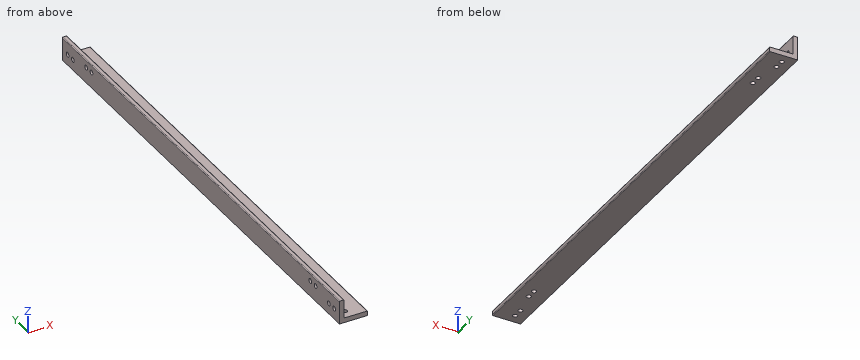
from build123d import *

# Parameters (mm, degrees)
SKETCH1_W           = 15
SKETCH1_H           = 313
SKETCH1_R           = 1.5
BOSS_EXTRUDE2_DEPTH = 3
SKETCH1_4_W         = 3
SKETCH1_4_H         = 313
BOSS_EXTRUDE3_DEPTH = 15
CUT_EXTRUDE1_REACH  = 20
SKETCH2_R           = 1.5
FILLET1_R           = 0.5


with BuildPart() as part:
    # Sketch1 → Boss-Extrude2 (new body)
    with BuildSketch(Plane.XY):
        with Locations((7.842857143, -137.142857143)):
            Rectangle(SKETCH1_W, SKETCH1_H)
        with Locations((4.142857143, 13.357142857)):
            Circle(SKETCH1_R, mode=Mode.SUBTRACT)
        with Locations((4.142857143, -287.642857143)):
            Circle(SKETCH1_R, mode=Mode.SUBTRACT)
        with Locations((4.142857143, 7.357142857)):
            Circle(SKETCH1_R, mode=Mode.SUBTRACT)
        with Locations((4.142857143, -281.642857143)):
            Circle(SKETCH1_R, mode=Mode.SUBTRACT)
        with Locations((7.342857143, -266.642857143)):
            Circle(SKETCH1_R, mode=Mode.SUBTRACT)
        with Locations((7.342857143, -260.642857143)):
            Circle(SKETCH1_R, mode=Mode.SUBTRACT)
        with Locations((7.342857143, -13.642857143)):
            Circle(SKETCH1_R, mode=Mode.SUBTRACT)
        with Locations((7.342857143, -7.642857143)):
            Circle(SKETCH1_R, mode=Mode.SUBTRACT)
    extrude(amount=BOSS_EXTRUDE2_DEPTH)

    # Sketch1_4 → Boss-Extrude3 (add)
    with BuildSketch(Plane.XY):
        with Locations((-1.157142857, -137.142857143)):
            Rectangle(SKETCH1_4_W, SKETCH1_4_H)
    extrude(amount=BOSS_EXTRUDE3_DEPTH)

    # Sketch2 → Cut-Extrude1 (cut, up to next)
    with BuildSketch(Plane.ZY.offset(2.657142857), mode=Mode.PRIVATE) as cut_extrude1_sk1:
        with Locations((6.8, 13.357142857)):
            Circle(SKETCH2_R)
    cut_extrude1_tool1 = extrude(cut_extrude1_sk1.sketch, amount=-CUT_EXTRUDE1_REACH, mode=Mode.PRIVATE) & part.part
    add(cut_extrude1_tool1.solids().sort_by_distance((-2.657143, 13.357143, 6.8))[0], mode=Mode.SUBTRACT)
    # Sketch2 → Cut-Extrude1 (cut, up to next)
    with BuildSketch(Plane.ZY.offset(2.657142857), mode=Mode.PRIVATE) as cut_extrude1_sk2:
        with Locations((6.8, -287.642857143)):
            Circle(SKETCH2_R)
    cut_extrude1_tool2 = extrude(cut_extrude1_sk2.sketch, amount=-CUT_EXTRUDE1_REACH, mode=Mode.PRIVATE) & part.part
    add(cut_extrude1_tool2.solids().sort_by_distance((-2.657143, -287.642857, 6.8))[0], mode=Mode.SUBTRACT)
    # Sketch2 → Cut-Extrude1 (cut, up to next)
    with BuildSketch(Plane.ZY.offset(2.657142857), mode=Mode.PRIVATE) as cut_extrude1_sk3:
        with Locations((6.8, -281.642857143)):
            Circle(SKETCH2_R)
    cut_extrude1_tool3 = extrude(cut_extrude1_sk3.sketch, amount=-CUT_EXTRUDE1_REACH, mode=Mode.PRIVATE) & part.part
    add(cut_extrude1_tool3.solids().sort_by_distance((-2.657143, -281.642857, 6.8))[0], mode=Mode.SUBTRACT)
    # Sketch2 → Cut-Extrude1 (cut, up to next)
    with BuildSketch(Plane.ZY.offset(2.657142857), mode=Mode.PRIVATE) as cut_extrude1_sk4:
        with Locations((6.8, 7.357142857)):
            Circle(SKETCH2_R)
    cut_extrude1_tool4 = extrude(cut_extrude1_sk4.sketch, amount=-CUT_EXTRUDE1_REACH, mode=Mode.PRIVATE) & part.part
    add(cut_extrude1_tool4.solids().sort_by_distance((-2.657143, 7.357143, 6.8))[0], mode=Mode.SUBTRACT)
    # Sketch2 → Cut-Extrude1 (cut, up to next)
    with BuildSketch(Plane.ZY.offset(2.657142857), mode=Mode.PRIVATE) as cut_extrude1_sk5:
        with Locations((10, -266.642857143)):
            Circle(SKETCH2_R)
    cut_extrude1_tool5 = extrude(cut_extrude1_sk5.sketch, amount=-CUT_EXTRUDE1_REACH, mode=Mode.PRIVATE) & part.part
    add(cut_extrude1_tool5.solids().sort_by_distance((-2.657143, -266.642857, 10))[0], mode=Mode.SUBTRACT)
    # Sketch2 → Cut-Extrude1 (cut, up to next)
    with BuildSketch(Plane.ZY.offset(2.657142857), mode=Mode.PRIVATE) as cut_extrude1_sk6:
        with Locations((10, -260.642857143)):
            Circle(SKETCH2_R)
    cut_extrude1_tool6 = extrude(cut_extrude1_sk6.sketch, amount=-CUT_EXTRUDE1_REACH, mode=Mode.PRIVATE) & part.part
    add(cut_extrude1_tool6.solids().sort_by_distance((-2.657143, -260.642857, 10))[0], mode=Mode.SUBTRACT)
    # Sketch2 → Cut-Extrude1 (cut, up to next)
    with BuildSketch(Plane.ZY.offset(2.657142857), mode=Mode.PRIVATE) as cut_extrude1_sk7:
        with Locations((10, -13.642857143)):
            Circle(SKETCH2_R)
    cut_extrude1_tool7 = extrude(cut_extrude1_sk7.sketch, amount=-CUT_EXTRUDE1_REACH, mode=Mode.PRIVATE) & part.part
    add(cut_extrude1_tool7.solids().sort_by_distance((-2.657143, -13.642857, 10))[0], mode=Mode.SUBTRACT)
    # Sketch2 → Cut-Extrude1 (cut, up to next)
    with BuildSketch(Plane.ZY.offset(2.657142857), mode=Mode.PRIVATE) as cut_extrude1_sk8:
        with Locations((10, -7.642857143)):
            Circle(SKETCH2_R)
    cut_extrude1_tool8 = extrude(cut_extrude1_sk8.sketch, amount=-CUT_EXTRUDE1_REACH, mode=Mode.PRIVATE) & part.part
    add(cut_extrude1_tool8.solids().sort_by_distance((-2.657143, -7.642857, 10))[0], mode=Mode.SUBTRACT)

    # Fillet1
    fillet1_edges = [part.edges().sort_by_distance(p)[0] for p in [
        (15.342857143, -137.142857143, 0),
        (0.342857143, -137.142857143, 15),
        (-2.657142857, -137.142857143, 15),
        (15.342857143, -137.142857143, 3),
        (0.342857143, -137.142857143, 3),
    ]]
    fillet(fillet1_edges, radius=FILLET1_R)


solid = part.part
Part model, mm, in its own coordinate system. Coordinates: 2 decimals unless noted, no trailing zeros. Write each loop counter-clockwise with the first axis right and the second up, starting at its lowest first coordinate (ties: lowest second). Pieces come first, ordered by that corner, then holes. Notation, with made-up numbers: M -21.75,56 L 19.25,56 A17 ccw 19.25,83 Z; hole C -29.75,48.25 d1. An arc over 180 degrees is marked long. Return JSON: item names as keys, results as strings.
1. Probe L1, parallel to Y at x = -1.7, z = 10; L2, parallel to Y at x = 6.75, z = 0.5; L3, parallel to X at y = -264.5, z = 10. List the from-to ranges inside material, lowest first.
Determined:
{"L1": "-293.64 to -268.14, -265.14 to -262.14, -259.14 to -15.14, -12.14 to -9.14, -6.14 to 19.36", "L2": "-293.64 to -268.02, -265.26 to -262.02, -259.26 to -15.02, -12.26 to -9.02, -6.26 to 19.36", "L3": "-2.66 to 0.34"}
2. Saw through at A-A, the plane y = -147. Write the cut outline in (x, z), then the cut area to 3 significant figures.
Determined:
{"outline": "M -2.66,0 L 14.84,0 A0.5 ccw 15.34,0.5 L 15.34,2.5 A0.5 ccw 14.84,3 L 0.84,3 A0.5 cw 0.34,3.5 L 0.34,14.5 A0.5 ccw -0.16,15 L -2.16,15 A0.5 ccw -2.66,14.5 Z", "area": "89.8 mm²"}
3. Flat gauge pins, fed straight in: pin 1 Ø4 at (y, z) = (-266.64, 10) entering from +X; pin 2 Ø1.5 at (x, z) = (3, 7) entering from -Y; pin 3 Ø8 at (x, z) = (7, 5) entering from +Y; pin 4 Ø1.5 at (x, y) = (1.5, -257) entering from +Z. Where does each tip first touch, or does it go through?
Determined:
{"pin 1": "x = 0.34", "pin 2": "through", "pin 3": "y = 19.36", "pin 4": "z = 3.01"}
